The listing builds one solid part. Answer for the finished solid, in the listing's coordinates (mm). Face numbers are marked on the shaded views. A direction names the side the tool comes from. Round coordinates to 2 decimals unless told otherwise and drop trailing zeros. Loops run counter-clockwise (first coordinate to the right, second up) from the corner with the lowest first, then second, coordinate; pieces in that order, holes last. Notation, with made-up numbers: (-1, -24.5) -> (28, -24.5) arc R7 ccw to (28, -18.5) -> close; hole circle Ø8 at (58.25, -33.5). An arc over 180 degrees is marked (long way). Use a Markdown table: item, result. Add a question column.
Q1. Section D-D on x = 32 is taken. Give the vertices of the cut face in (y, z), then the cut area to 3 significant figures.
Q2. Section B-B on z = 28 is taken. Give the number of separate pieces and of enclosed holes in the cut face, then the cut area to 4 significant figures.
Q3. Which of the six approach directions +Z, -Z, +X, -X, +Y, -Y give full straight-line access (tool end or side, diameter ignored) to the marked faces 5 and 6?
Q4. Section A-A on y = 61 is taken. Give the vertices of the cut face in (x, z), then the cut area to 3 significant figures.
Q5. Consider line 1 (X direction, y = 40, z = 26); line 2 (Y direction, x = 72.5, z = 15.5); line 3 (Y direction, x = 43.5, z = 7.5). Determine where each line is inside the solid, lowest interval first.
Q6. For a pull along Y with two mould halves and no side action, classify the marked faces 1, 2, 3 and 4 as released by +Y, released by -Y, zero draft, split by the parting line, or undercut.
Q7. Given pin 1 Ø4 at (y, z) = (42, 7.5) entering from -X; pin 2 Ø12 at (x, y) = (81, 59.5) entering from -Z; pin 3 Ø2.5 at (y, z) = (35, 37) entering from -X; pin 4 Ø5.5 at (x, y) = (3, 62.5) entering from -Z, each flat-ended and moving along its own axis, determine where each tip first touches the part or whether it passes through.
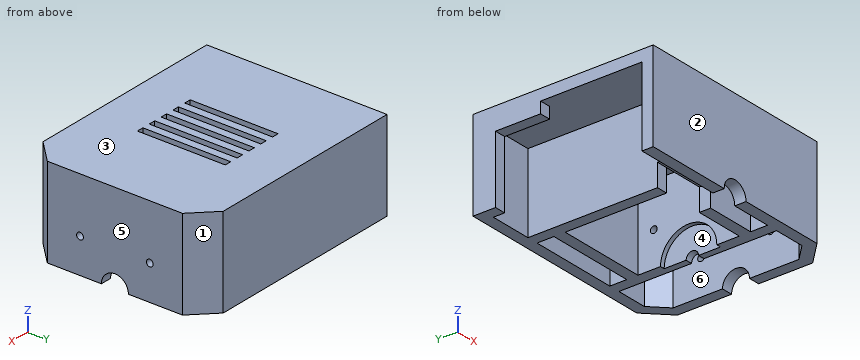
Autodesk Inventor part; units mm, degrees
ref_plane "YZ Plane" through (0, 0, 0) normal (1, 0, 0) x (0, 1, 0)
ref_plane "XZ Plane" through (0, 0, 0) normal (0, 1, 0) x (-1, 0, 0)
ref_plane "XY Plane" through (0, 0, 0) normal (0, 0, 1) x (1, 0, 0)
sketch "Sketch1" plane through (0, 0, 0) normal (0, 0, 1) x (1, 0, 0)
  line L0 (0, 0) -> (100, 0)
  line L1 (100, 0) -> (100, 80) construction
  line L2 (100, 80) -> (0, 80)
  line L3 (0, 80) -> (0, 0)
  line L4 (100, 70) -> (90, 80)
  line L5 (100, 10) -> (90, 0)
  line L6 (100, 70) -> (100, 10)
  dimension "d0" = 100
  dimension "d1" = 80
  dimension "d23" = 10
  dimension "d24" = 10
  dimension "d25" = 10
  dimension "d26" = 10
extrude "Extrusion1" add sketch "Sketch1" along normal blind 40
sketch "Sketch4" plane through (0, 0, 0) normal (0, 0, -1) x (-1, 0, 0)
  line L0 (-90, 80) -> (0, 80)
  line L1 (0, 0) -> (-90, 0)
  line L2 (-100, 70) -> (-90, 80)
  line L3 (-100, 10) -> (-100, 70)
  line L4 (-90, 0) -> (-100, 10)
  line L5 (0, 75) -> (-87.9289, 75)
  line L6 (-87.9289, 75) -> (-95, 67.9289)
  line L7 (-95, 67.9289) -> (-95, 12.0711)
  line L8 (-95, 12.0711) -> (-87.9289, 5)
  line L9 (-87.9289, 5) -> (0, 5)
  line L10 (0, 75) -> (0, 5)
  line L11 (0, 80) -> (0, 0)
  dimension "d27" = 5
extrude "Extrusion4" cut sketch "Sketch4" against normal blind 35 contours L10 L9 L8 L7 L6 L5
sketch "Sketch5" plane through (0, 0, 40) normal (-1, 0, 0) x (0, 0, 1)
  line L0 (0, 0) -> (0, 80)
  line L1 (-40, 5) -> (-40, 75)
  line L2 (0, 80) -> (-40, 80)
  line L3 (-40, 80) -> (-40, 70)
  line L4 (-40, 70) -> (0, 70)
  line L5 (0, 70) -> (0, 80)
  line L6 (0, 80) -> (-10, 80)
  line L7 (-10, 80) -> (-10, 50)
  line L8 (-10, 50) -> (0, 50)
  line L9 (0, 50) -> (0, 80)
  line L10 (-40, 0) -> (0, 0)
  dimension "d15" = 10
  dimension "d16" = 10
  dimension "d17" = 50
extrude "Extrusion5" add sketch "Sketch5" against normal blind 5
sketch "Sketch6" plane through (100, 10, 0) normal (1, 0, 0) x (0, 0, -1)
  circle A0 centre (0, 30) radius 6
  line L0 (0, 0) -> (0, 60)
  dimension "d20" = 12
extrude "Extrusion6" cut sketch "Sketch6" against normal through all
sketch "Sketch7" plane through (0, 0, 35) normal (0, 0, -1) x (-1, 0, 0)
  line L0 (-87.9289, 75) -> (-5, 75)
  line L1 (0, 5) -> (-87.9289, 5)
  line L2 (-74, 75) -> (-69, 75)
  line L3 (-69, 75) -> (-69, 5)
  line L4 (-69, 5) -> (-74, 5)
  line L5 (-74, 5) -> (-74, 75)
  line L6 (-95, 46) -> (-95, 67.9289)
  line L7 (-29, 75) -> (-24, 75)
  line L8 (-24, 75) -> (-24, 5)
  line L9 (-24, 5) -> (-29, 5)
  line L10 (-29, 5) -> (-29, 75)
  line L11 (-69, 67.5) -> (-29, 67.5)
  line L12 (-29, 67.5) -> (-29, 62.5)
  line L13 (-29, 62.5) -> (-69, 62.5)
  line L14 (-69, 62.5) -> (-69, 67.5)
  line L15 (-69, 17.5) -> (-29, 17.5)
  line L16 (-29, 17.5) -> (-29, 12.5)
  line L17 (-29, 12.5) -> (-69, 12.5)
  line L18 (-69, 12.5) -> (-69, 17.5)
  line L19 (-49, 67.5) -> (-49, 12.5) construction
  point P0 (0, 0)
  point P1 (-49, 40)
  point P2 (-69, 40)
  dimension "d28" = 5
  dimension "d29" = 21
  dimension "d30" = 5
  dimension "d31" = 40
  dimension "d32" = 5
  dimension "d33" = 5
  dimension "d34" = 45
extrude "Extrusion7" add sketch "Sketch7" along normal blind 35 contours L0 L3 L1 L5 | L0 L8 L1 L10 | L11 L10 L13 L3 | L3 L15 L10 L17
sketch "Sketch8" plane through (0, 0, 0) normal (0, 0, -1) x (-1, 0, 0)
  line L0 (-24, 5) -> (-24, 75)
  line L1 (-69, 17.5) -> (-29, 17.5)
  line L2 (-24, 5) -> (-47, 5)
  line L3 (-47, 5) -> (-47, 17.5)
  line L4 (-47, 17.5) -> (-24, 17.5)
  line L5 (-24, 17.5) -> (-24, 5)
  point P0 (0, 0)
  dimension "d37" = 23
extrude "Extrusion8" cut sketch "Sketch8" against normal blind 10
sketch "Sketch9" plane through (69, 17.5, 35) normal (-1, 0, 0) x (0, 0, 1)
  line L0 (-35, 0) -> (-35, 45)
  circle A0 centre (-35, 22.5) radius 2.75
  line L1 (-50.5, 7) -> (-19.5, 7) construction
  line L2 (-19.5, 7) -> (-19.5, 38) construction
  line L3 (-19.5, 38) -> (-50.5, 38) construction
  line L4 (-50.5, 38) -> (-50.5, 7) construction
  line L5 (-50.5, 7) -> (-19.5, 38) construction
  line L6 (-19.5, 7) -> (-50.5, 38) construction
  circle A1 centre (-19.5, 38) radius 1.5
  circle A2 centre (-19.5, 7) radius 1.5
  point P0 (-35, -17.5)
  dimension "d40" = 5.5
  dimension "d41" = 31
  dimension "d42" = 31
  dimension "d43" = 3
  dimension "d44" = 3
extrude "Extrusion9" cut sketch "Sketch9" against normal through all
sketch "Sketch10" plane through (0, 0, 35) normal (0, 0, -1) x (-1, 0, 0)
  line L0 (-34.5, 59.5) -> (-37.5, 59.5)
  line L1 (-37.5, 59.5) -> (-37.5, 20.5)
  line L2 (-37.5, 20.5) -> (-34.5, 20.5)
  line L3 (-34.5, 20.5) -> (-34.5, 59.5)
  line L4 (-29, 62.5) -> (-29, 17.5)
  line L5 (-69, 62.5) -> (-29, 62.5)
  line L6 (-29, 17.5) -> (-24, 17.5)
  line L7 (-41, 59.5) -> (-44, 59.5)
  line L8 (-44, 59.5) -> (-44, 20.5)
  line L9 (-44, 20.5) -> (-41, 20.5)
  line L10 (-41, 20.5) -> (-41, 59.5)
  line L11 (-47.5, 59.5) -> (-50.5, 59.5)
  line L12 (-50.5, 59.5) -> (-50.5, 20.5)
  line L13 (-50.5, 20.5) -> (-47.5, 20.5)
  line L14 (-47.5, 20.5) -> (-47.5, 59.5)
  line L15 (-54, 59.5) -> (-57, 59.5)
  line L16 (-57, 59.5) -> (-57, 20.5)
  line L17 (-57, 20.5) -> (-54, 20.5)
  line L18 (-54, 20.5) -> (-54, 59.5)
  line L19 (-60.5, 59.5) -> (-63.5, 59.5)
  line L20 (-63.5, 59.5) -> (-63.5, 20.5)
  line L21 (-63.5, 20.5) -> (-60.5, 20.5)
  line L22 (-60.5, 20.5) -> (-60.5, 59.5)
  point P0 (0, 0)
  dimension "d47" = 3
  dimension "d49" = 5.5
  dimension "d50" = 3
  dimension "d51" = 3
  dimension "d54" = 6.5
extrude "Extrusion10" cut sketch "Sketch10" against normal through all
sketch "Sketch11" plane through (0, 0, 0) normal (0, -1, 0) x (1, 0, 0)
  circle A0 centre (45, 0) radius 6
  line L0 (0, 0) -> (90, 0)
  dimension "d61" = 12
extrude "Extrusion11" cut sketch "Sketch11" against normal blind 5
sketch "Sketch12" plane through (69, 17.5, 35) normal (-1, 0, 0) x (0, 0, 1)
  arc A0 (-35, 19.75) -> (-35, 25.25) centre (-35, 22.5) ccw
  circle A1 centre (-35, 22.5) radius 12.5
  point P0 (-35, -17.5)
  dimension "d64" = 25
extrude "Extrusion12" cut sketch "Sketch12" against normal blind 2
properties part number "FA002" material "ABS Plastic"
Checked values:
| question | item | result |
|---|---|---|
| 1 | outline | (0, 0) -> (5, 0) -> (5, 35) -> (12.5, 35) -> (12.5, 10) -> (17.5, 10) -> (17.5, 35) -> (62.5, 35) -> (62.5, 0) -> (67.5, 0) -> (67.5, 35) -> (75, 35) -> (75, 0) -> (80, 0) -> (80, 40) -> (0, 40) -> close |
| 1 | area | 1,050 mm2 |
| 2 | separate pieces | 1 |
| 2 | enclosed holes | 4 |
| 2 | area | 2,425 mm2 |
| 3 | face 5 | +Z, -Z, +X, +Y, -Y |
| 3 | face 6 | -Z |
| 4 | outline | (0, 30) -> (5, 30) -> (5, 35) -> (24, 35) -> (24, 0) -> (29, 0) -> (29, 35) -> (69, 35) -> (69, 0) -> (74, 0) -> (74, 35) -> (95, 35) -> (95, 0) -> (100, 0) -> (100, 40) -> (0, 40) -> close |
| 4 | area | 1,050 mm2 |
| 5 | line 1 | x = 24 to 29, 69 to 74, 95 to 100 |
| 5 | line 2 | y = 0 to 23, 26 to 54, 57 to 80 |
| 5 | line 3 | y = 0 to 5, 62.5 to 67.5, 75 to 80 |
| 6 | face 1 | released by +Y |
| 6 | face 2 | released by -Y |
| 6 | face 3 | zero draft |
| 6 | face 4 | undercut |
| 7 | pin 1 | stops at x = 24 |
| 7 | pin 2 | stops at z = 35 |
| 7 | pin 3 | stops at x = 0 |
| 7 | pin 4 | stops at z = 30 |
